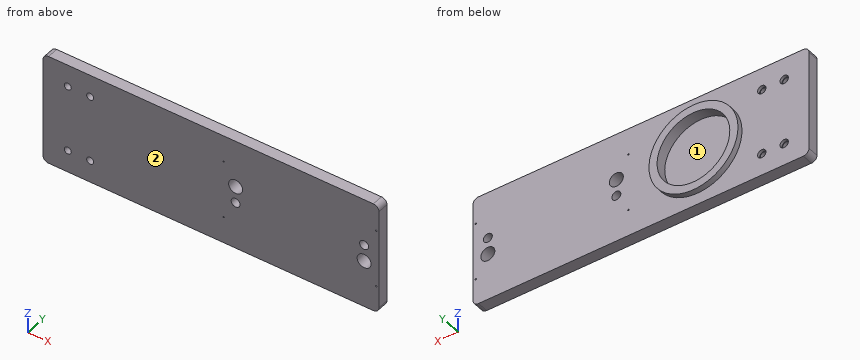
```python
from build123d import *

# Parameters (mm, degrees)
SKETCH1_W           = 600
SKETCH1_H           = 200
BOSS_EXTRUDE1_DEPTH = 20
SKETCH2_R           = 6.25
CUT_EXTRUDE1_DEPTH  = 633.771680782
SKETCH4_R           = 7.5
CUT_EXTRUDE2_DEPTH  = 5
SKETCH5_R           = 1.25
CUT_EXTRUDE3_DEPTH  = 633.771680782
FILLET1_R           = 10
SKETCH6_R           = 79.491583248
BOSS_EXTRUDE2_DEPTH = 10
SKETCH7_R           = 64.936608028
CUT_EXTRUDE4_DEPTH  = 19
SKETCH8_R           = 12.5
SKETCH8_R_2         = 8
CUT_EXTRUDE5_DEPTH  = 633.771680782


with BuildPart() as part:
    # Sketch1 → Boss-Extrude1 (new body)
    with BuildSketch(Plane(origin=(0, 0, 0), x_dir=(1, 0, 0), z_dir=(0, 1, 0))):
        with Locations((-300, 100)):
            Rectangle(SKETCH1_W, SKETCH1_H)
    extrude(amount=BOSS_EXTRUDE1_DEPTH)

    # Sketch2 → Cut-Extrude1 (cut, through all)
    with BuildSketch(Plane(origin=(0, 20, 0), x_dir=(1, 0, 0), z_dir=(0, 1, 0))):
        with Locations(Location((-555.774, 160, 0), (0, 0, 270))):
            Circle(SKETCH2_R)
        with Locations(Location((-555.774, 40, 0), (0, 0, 270))):
            Circle(SKETCH2_R)
        with Locations(Location((-515.774, 40, 0), (0, 0, 90))):
            Circle(SKETCH2_R)
        with Locations(Location((-515.774, 160, 0), (0, 0, 90))):
            Circle(SKETCH2_R)
    extrude(amount=-CUT_EXTRUDE1_DEPTH, mode=Mode.SUBTRACT)

    # Sketch4 → Cut-Extrude2 (cut)
    with BuildSketch(Plane(origin=(0, 20, 0), x_dir=(1, 0, 0), z_dir=(0, 1, 0))):
        with Locations(Location((-555.774, 160, 0), (0, 0, 270))):
            Circle(SKETCH4_R)
        with Locations(Location((-555.774, 40, 0), (0, 0, 270))):
            Circle(SKETCH4_R)
        with Locations(Location((-515.774, 40, 0), (0, 0, 90))):
            Circle(SKETCH4_R)
        with Locations(Location((-515.774, 160, 0), (0, 0, 90))):
            Circle(SKETCH4_R)
    extrude(amount=-CUT_EXTRUDE2_DEPTH, mode=Mode.SUBTRACT)

    # Sketch5 → Cut-Extrude3 (cut, through all)
    with BuildSketch(Plane(origin=(0, 20, 0), x_dir=(1, 0, 0), z_dir=(0, 1, 0))):
        with Locations(Location((-277.5, 48, 0), (0, 0, 270))):
            Circle(SKETCH5_R)
        with Locations(Location((-277.5, 152, 0), (0, 0, 90))):
            Circle(SKETCH5_R)
        with Locations(Location((-5, 48, 0), (0, 0, 90))):
            Circle(SKETCH5_R)
        with Locations(Location((-5, 152, 0), (0, 0, 270))):
            Circle(SKETCH5_R)
    extrude(amount=-CUT_EXTRUDE3_DEPTH, mode=Mode.SUBTRACT)

    # Fillet1
    fillet1_edges = [part.edges().sort_by_distance(p)[0] for p in [
        (0, 10, 0),
        (-600, 10, 0),
        (-600, 10, -200),
        (0, 10, -200),
    ]]
    fillet(fillet1_edges, radius=FILLET1_R)

    # Sketch6 → Boss-Extrude2 (add)
    with BuildSketch(Plane(origin=(0, 20, 0), x_dir=(1, 0, 0), z_dir=(0, 1, 0))):
        with Locations(Location((-400.867107023, 100, 0), (0, 0, 270))):
            Circle(SKETCH6_R)
    extrude(amount=BOSS_EXTRUDE2_DEPTH)

    # Sketch7 → Cut-Extrude4 (cut)
    with BuildSketch(Plane(origin=(0, 30, 0), x_dir=(1, 0, 0), z_dir=(0, 1, 0))):
        with Locations(Location((-400.867107023, 100, 0), (0, 0, 270))):
            Circle(SKETCH7_R)
    extrude(amount=-CUT_EXTRUDE4_DEPTH, mode=Mode.SUBTRACT)

    # Sketch8 → Cut-Extrude5 (cut, through all)
    with BuildSketch(Plane(origin=(0, 20, 0), x_dir=(1, 0, 0), z_dir=(0, 1, 0))):
        with Locations(Location((-26.5, 115, 0), (0, 0, 270))):
            Circle(SKETCH8_R)
        with Locations(Location((-26.5, 85, 0), (0, 0, 270))):
            Circle(SKETCH8_R_2)
        with Locations(Location((-256, 115, 0), (0, 0, 270))):
            Circle(SKETCH8_R_2)
        with Locations(Location((-256, 85, 0), (0, 0, 270))):
            Circle(SKETCH8_R)
    extrude(amount=-CUT_EXTRUDE5_DEPTH, mode=Mode.SUBTRACT)


solid = part.part
```
CAD build for the part. Positions are in the model's coordinates, mm. Face numbers are marked on the shaded views. Coordinates: 2 decimals unless noted, no trailing zeros. Write each loop counter-clockwise with the first axis right and the second up, starting at its lowest first coordinate (ties: lowest second). Pieces come first, ordered by that corner, then holes.
(1) Cut at D-D, the plane x = -371.5. List the corners of the cut face in (y, z), and give its area (3 significant figures).
(2) Two-plate mould, pull along Z, no slides. Class the marked faces 1 and 2: +Z half, -Z half, draft (parallel to the pull), parting line (faces both ways), or undercut.
(3) Drill centre lines: probe 1 along Z at (x, y) = (-277.5, 5.5); probe 2 along X at (y, z) = (9.75, -160); probe 3 along X at (y, z) = (17.65, -40). Where is each one in solid material? Low to high.
(4) Cut at A-A, the plane x = -256. List the corners of the cut face in (y, z), and give its area (3 significant figures).
(5) Cut at C-C, the plane x = -489. List the corners of the cut face in (y, z).
(6) Flat gauge pins, fed straight in: pin 1 (3 mm diameter, centred on x = -220, z = -23.5, fed in from +Y); pin 2 (2 mm diameter, centred on x = -433, z = -66.5, fed in from +Y); pin 3 (13.5 mm diameter, centred on x = -555.774, z = -160, fed in from +Y). Where does each tip first touch, or does it go through?
(7) Cut at B-B, the plane z = -115. List the corners of the cut face in (x, y), and give its area (3 significant figures).
Geometry says:
1. outline: (0, -200) - (20, -200) - (20, -173.87) - (30, -173.87) - (30, -157.92) - (11, -157.92) - (11, -42.08) - (30, -42.08) - (30, -26.13) - (20, -26.13) - (20, 0) - (0, 0) - close
1. area: 3,280 mm2
2. face 1: undercut
2. face 2: draft
3. probe 1: z = -200 to -153.25, -150.75 to -49.25, -46.75 to 0
3. probe 2: x = -600 to -562.02, -549.52 to -522.02, -509.52 to 0
3. probe 3: x = -600 to -563.27, -548.27 to -523.27, -508.27 to -425.7, -376.03 to 0
4. outline: (0, -200) - (20, -200) - (20, -123) - (0, -123) - close; (0, -107) - (20, -107) - (20, -97.5) - (0, -97.5) - close; (0, -72.5) - (20, -72.5) - (20, 0) - (0, 0) - close
4. area: 3,180 mm2
5. outline: (0, -200) - (20, -200) - (20, 0) - (0, 0) - close
6. pin 1: stops at y = 20
6. pin 2: stops at y = 11
6. pin 3: stops at y = 15
7. outline: (-600, 0) - (-264, 0) - (-264, 20) - (-322.8, 20) - (-322.8, 30) - (-337.69, 30) - (-337.69, 11) - (-464.05, 11) - (-464.05, 30) - (-478.93, 30) - (-478.93, 20) - (-600, 20) - close; (-248, 0) - (-39, 0) - (-39, 20) - (-248, 20) - close; (-14, 0) - (0, 0) - (0, 20) - (-14, 20) - close
7. area: 10,300 mm2
